from build123d import *

# Parameters (mm, degrees)
F0_W      = 50.8
F0_H      = 50.8
F1_DEPTH  = 25.4
F1_FACE_W = 50.8
F1_FACE_H = 50.8
F2_DEPTH  = 101.6
F3_R      = 38.1
F4_DEPTH  = 304.8
F5_R      = 38.1


with BuildPart() as f1:
    # F0 (on Front) → F1 (new body)
    with BuildSketch(Plane.XZ):
        Rectangle(F0_W, F0_H)
    extrude(amount=F1_DEPTH)

    # F1_face (on face) → F2 (join)
    with BuildSketch(Plane.XZ.offset(25.4)):
        Rectangle(F1_FACE_W, F1_FACE_H)
    extrude(amount=F2_DEPTH)

    # F3 (on face) → F4 (join)
    with BuildSketch(Plane.XZ.offset(127)):
        Circle(F3_R)
    extrude(amount=F4_DEPTH)

    # F5
    f5_edges = [f1.edges().sort_by_distance(p)[0] for p in [
        (-38.1, -431.8, 0),
    ]]
    fillet(f5_edges, radius=F5_R)


solid = f1.part
Input: part model. Units: mm. Frame: model coordinates. A direction names the side the tool comes from. Give positions to 0.01 mm unless a question says otherwise; leave off trailing zeros. Order: outer loops, then holes, each group sorted by start corner. A loop starts at its lowest first (then second) coordinate and runs counter-clockwise, first axis right, second up. Notation, with made-up numbers: M 77.5,-36 L 126.5,-36 A26 cw 126.5,-2 Z; hole C -31.5,85 d4. An arc over 180 degrees is marked long. Answer as a JSON object with one key per item and string values.
1. Ray query, line 1 (X direction, y = -46.5, z = 4); line 2 (Z direction, x = -2, y = -180.5). Return the intervals inside material, ascending. Write a range as [from, to].
Result sheet:
{"line 1": "[-25.4, 25.4]", "line 2": "[-38.05, 38.05]"}
2. Reachability of faces 1 (the flat face through (25.4, -63, 0)), 2 (the flat face through (0, -63, 25.4)), 3 (the flat face through (0, -63, -25.4)), 4 (the flat face through (-25.4, -63, 0)), 5 (the cylindrical face through (-30.235, -258.483, -23.183)) from +Z, -Z, +X, -X, +Y, -Y: full face, straight path, thin tool, end or side. Return the list, or none.
Result sheet:
{"face 1": "+Z, -Z, +X, +Y", "face 2": "+Z, +X, -X, +Y", "face 3": "-Z, +X, -X, +Y", "face 4": "+Z, -Z, -X, +Y", "face 5": "+Y, -Y"}
3. Cut plane A-A, the plane x = 0. Output: boundary loops of the cut face in (y, z), and give its area (3 significant figures).
Result sheet:
{"outline": "M -393.7,-38.1 L -127,-38.1 L -127,-25.4 L 0,-25.4 L 0,25.4 L -127,25.4 L -127,38.1 L -393.7,38.1 A38.1 ccw Z", "area": "29,100 mm²"}
4. Cut plane B-B, the plane z = 0. Output: boundary loops of the cut face in (x, y), and give its area (3 significant figures).
Result sheet:
{"outline": "M -38.1,-393.7 A38.1 ccw 38.1,-393.7 L 38.1,-127 L 25.4,-127 L 25.4,0 L -25.4,0 L -25.4,-127 L -38.1,-127 Z", "area": "29,100 mm²"}
5. Cut plane C-C, the plane y = -114. Output: boundary loops of the cut face in (x, z), and give its area (3 significant figures).
Result sheet:
{"outline": "M -25.4,-25.4 L 25.4,-25.4 L 25.4,25.4 L -25.4,25.4 Z", "area": "2,580 mm²"}
6. First-contact query: P1, Ø15, axis at x = 2, y = -80.5, coming from the +Z side; P2, Ø10, axis at x = 13.5, z = -14, coming from the -Y side; P3, Ø10, axis at x = 4, y = -270.5, coming from the +Z side. Flat tips, straight axial feed; report the tip coordinate or a pass-through.
Result sheet:
{"P1": "z = 25.4", "P2": "y = -428.95", "P3": "z = 38.1"}
7. Cut plane D-D, the plane y = -172.5. Output: boundary loops of the cut face in (x, z).
Result sheet:
{"outline": "C 0,0 d76.2"}
